from build123d import *

# Parameters (mm, degrees)
SKETCH1_W           = 210
SKETCH1_H           = 150
BOSS_EXTRUDE1_DEPTH = 10
SKETCH2_W           = 120
SKETCH2_H           = 105
CUT_EXTRUDE1_DEPTH  = 2
SKETCH3_R           = 4
CUT_EXTRUDE2_DEPTH  = 5


with BuildPart() as part:
    # Sketch1 → Boss-Extrude1 (new body)
    with BuildSketch(Plane.XY):
        Rectangle(SKETCH1_W, SKETCH1_H)
    extrude(amount=BOSS_EXTRUDE1_DEPTH)

    # Sketch2 → Cut-Extrude1 (cut)
    with BuildSketch(Plane.XY.offset(10)):
        Rectangle(SKETCH2_W, SKETCH2_H)
    extrude(amount=-CUT_EXTRUDE1_DEPTH, mode=Mode.SUBTRACT)

    # Sketch3 → Cut-Extrude2 (cut)
    with BuildSketch(Plane(origin=(0, 75, 0), x_dir=(1, 0, 0), z_dir=(0, 1, 0))):
        with Locations(Location((-9.942757001, -5, 0), (0, 0, 270))):
            Circle(SKETCH3_R)
        with Locations(Location((9.942757001, -5, 0), (0, 0, 90))):
            Circle(SKETCH3_R)
    extrude(amount=-CUT_EXTRUDE2_DEPTH, mode=Mode.SUBTRACT)


solid = part.part
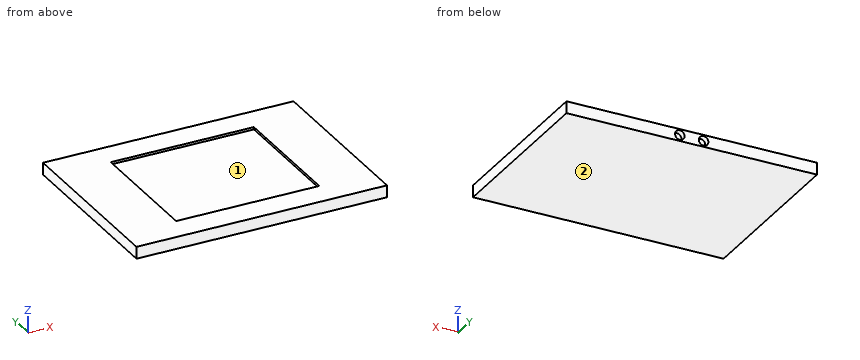
Build history of the part. All positions in model axes, mm. Face numbers are marked on the shaded views. Round coordinates to 2 decimals unless told otherwise and drop trailing zeros. Write each loop counter-clockwise with the first axis right and the second up, starting at its lowest first coordinate (ties: lowest second). Pieces come first, ordered by that corner, then holes. Notation, with made-up numbers: (-33.5, 53.25) -> (15.5, 53.25) arc R16 cw to (15.5, 68.25) -> close; hole circle Ø10 at (49.25, 32). An arc over 180 degrees is marked (long way). Use one line per item in the form item = value.
Q1. Band-saw the part on B-B, the plane x = -35.5. Write the cut outline in (y, z).
Conclusion:
outline = (-75, 0) -> (75, 0) -> (75, 10) -> (52.5, 10) -> (52.5, 8) -> (-52.5, 8) -> (-52.5, 10) -> (-75, 10) -> close
Q2. Drop a flat-ended pin along its axis: P1, Ø4, axis at x = -11, z = 5.5, coming from the +Y side. Give the stop position or say it passes through.
Conclusion:
P1 = 70
Q3. Drill centre lines: L1, parallel to X at y = 71.65, z = 5; L2, parallel to Y at x = -57.5, z = 8.5; L3, parallel to X at y = 36, z = 8.75. Where is each one in solid material? Low to high.
Conclusion:
L1 = -105 to -13.94, -5.94 to 5.94, 13.94 to 105
L2 = -75 to -52.5, 52.5 to 75
L3 = -105 to -60, 60 to 105
Q4. Band-saw the part on A-A, the plane y = -46.5. Write the cut outline in (x, z), then the cut area to 3 significant figures.
Conclusion:
outline = (-105, 0) -> (105, 0) -> (105, 10) -> (60, 10) -> (60, 8) -> (-60, 8) -> (-60, 10) -> (-105, 10) -> close
area = 1,860 mm²
Q5. Two-plate mould, pull along X, no slides. Class the marked faces 1 and 2: released by +X, released by -X, zero draft, split by the parting line, or undercut.
Conclusion:
face_1 = undercut
face_2 = zero draft
